Build history of the part. All positions in model axes, mm. A direction names the side the tool comes from. Round coordinates to 2 decimals unless told otherwise and drop trailing zeros. Write each loop counter-clockwise with the first axis right and the second up, starting at its lowest first coordinate (ties: lowest second). Pieces come first, ordered by that corner, then holes.
Item 1: Mould opens along Y. For faces 1 (the cylindrical face through (51.1, -28.24, 52.61)), 2 (the flat face through (74, -49, 100)), 3 (the flat face through (51, -100, 51)) say: +Y half, -Y half, draft (parallel to the pull), parting line (faces both ways), or undercut.
Item 2: Band-saw the part on C-C, the plane x = 89. Write the cut outline in (y, z), then the cut area to 3 significant figures.
Item 3: Drop flat-ended pins along their axis: pin 1 Ø1.5 at (x, y) = (92, -22.5) entering from -Z; pin 2 Ø12 at (x, y) = (69, -10) entering from +Z; pin 3 Ø2 at (y, z) = (-68.5, -24) entering from +X; pin 4 Ø5 at (x, z) = (60, 66) entering from +Y. Give the stop position or say it passes through.
Item 4: Wall check: probe 1 along Y at (x, z) = (7.5, 50); probe 2 along Z at (x, y) = (26.5, -34.5); probe 3 along Z at (x, y) = (45.5, -82). Give the ranges that are in metal, low to high.
Item 5: Band-saw the part on A-A, the plane y = -56. Write the cut outline in (x, z).
Item 6: 3-axis set-ups, long thin cutter, end or side, ignore diameter. For faces 4 (the flat face through (63, -27, 0)), 5 (the cylindrical face through (23.65, -49.78, 124.65)), 6 (the flat face through (0, -27, 49)): which of +Z, -Z, +X, -X, +Y, -Y reach the whole face in a straight line?
Item 7: Band-saw the part on B-B, the plane z = 74. Write the cut outline in (x, y), then the cut area to 3 significant figures.
Item 8: Band-saw the part on D-D, the plane y = -18.5. Write the cut outline in (x, z), then the cut area to 3 significant figures.
```python
from build123d import *

# Parameters (mm, degrees)
F1_W     = 103.645719
F1_H     = 100
F2_DEPTH = 100
F6_D     = 50
F3_R     = 25
F7_DEPTH = 50
F4_R     = 25
F8_DEPTH = 50


with BuildPart() as f2:
    # F1 (on face) → F2 (new body)
    with BuildSketch(Plane.XZ):
        with Locations((51.822859, 50)):
            Rectangle(F1_W, F1_H)
    extrude(amount=F2_DEPTH)

    # F6 (through all)
    with Locations(Plane.YZ.offset(103.645719)):
        with Locations((-53.215325, 51.51242)):
            Hole(F6_D / 2)

    # F3 (on face) → F7 (join)
    with BuildSketch(Plane.XY.offset(100)):
        with Locations((48.626781, -50.881982)):
            Circle(F3_R)
    extrude(amount=F7_DEPTH)

    # F4 (on face) → F8 (join)
    with BuildSketch(Plane(origin=(0, 0, 0), x_dir=(1, 0, 0), z_dir=(0, 0, -1))):
        with Locations((49.750507, 50.30711)):
            Circle(F4_R)
    extrude(amount=F8_DEPTH)


solid = f2.part
```
Results:
1. face 1: undercut
1. face 2: draft
1. face 3: -Y half
2. outline: (-100, 0) - (0, 0) - (0, 100) - (-100, 100) - close; hole circle Ø50 at (-53.22, 51.51)
2. area: 8,040 mm2
3. pin 1: stops at z = 0
3. pin 2: stops at z = 100
3. pin 3: stops at x = 67.9
3. pin 4: stops at y = 0
4. probe 1: y = -100 to -78.17, -28.26 to 0
4. probe 2: z = 0 to 34.94, 68.09 to 100
4. probe 3: z = 0 to 100
5. outline: (0, 0) - (25.41, 0) - (25.41, -50) - (74.09, -50) - (74.09, 0) - (103.65, 0) - (103.65, 26.67) - (0, 26.67) - close; (0, 76.36) - (103.65, 76.36) - (103.65, 100) - (73.1, 100) - (73.1, 150) - (24.16, 150) - (24.16, 100) - (0, 100) - close
6. face 4: -Z
6. face 5: +Z
6. face 6: +Z, -Z, -X, +Y, -Y
7. outline: (0, -100) - (103.65, -100) - (103.65, -64.14) - (0, -64.14) - close; (0, -42.29) - (103.65, -42.29) - (103.65, 0) - (0, 0) - close
7. area: 8,100 mm2
8. outline: (0, 0) - (103.65, 0) - (103.65, 100) - (0, 100) - close
8. area: 10,400 mm2
